Design review of the part built by this model. Coordinates are the model's own, in mm. Give positions to 0.01 mm unless a question says otherwise; leave off trailing zeros. Loops run counter-clockwise (first coordinate to the right, second up) from the corner with the lowest first, then second, coordinate; pieces in that order, holes last. Notation, with made-up numbers: M 4.5,24.5 L 55.5,24.5 A16 ccw 55.5,35.5 Z; hole C 10.5,61 d10. An arc over 180 degrees is marked long. Use a Markdown table: item, result. Add a question column.
(1) Insertion check: pin 1 Ø8 at (x, z) = (-42.5, -36.5) entering from +Y; pin 2 Ø8 at (y, z) = (-12.5, -1.5) entering from -X; pin 3 Ø4 at (y, z) = (-2, 41.5) entering from +X; pin 4 Ø5 at (x, z) = (-48, 65) entering from -Y. Each pin has a flat end and moves straight along its axis. Give the tip position at first contact, or say it passes through.
(2) For probe 1 along Z at (x, y) = (-10, -3); probe 2 along Z at (x, y) = (63, -2); probe 3 along X at (y, z) = (-17, -75), list the stretches that pass through material, from the lowest coordinate up.
(3) Add section C-C, the plane z = 24. Give the boundary of the cut face in (x, y), then the cut area to 3 significant figures.
(4) Add section A-A, the plane y = -20.25. Give the boundary of the cut face in (x, z), then the cut area to 3 significant figures.
(5) Add section D-D, the plane x = 24. Give the boundary of the cut face in (y, z).
```python
from build123d import *

# Parameters (mm, degrees)
SKETCH1_W            = 5.08
SKETCH1_H            = 5.08
BOSS_EXTRUDE2_DEPTH  = 5.08
BOSS_EXTRUDE7_DEPTH  = 5.08
BOSS_EXTRUDE8_DEPTH  = 1.27
BOSS_EXTRUDE9_DEPTH  = 12.7
BOSS_EXTRUDE10_DEPTH = 12.7
SKETCH1_5_W          = 5.08
SKETCH1_5_H          = 5.08
BOSS_EXTRUDE12_DEPTH = 25.4
BOSS_EXTRUDE13_DEPTH = 2.54
FILLET4_R            = 5.08


with BuildPart() as part:
    # Sketch1 → Boss-Extrude2 (new body)
    with BuildSketch(Plane(origin=(0, 0, 0), x_dir=(1, 0, 0), z_dir=(0, 1, 0))):
        Polygon((1.79979496, -9.735410081), (75.45979496, -9.735410081), (75.45979496, 85.514589919), (-19.79020504, 85.514589919), (-19.79020504, 34.079589919), (18.30979496, 34.079589919), (19.57979496, 34.079589919), (24.02479496, 34.079589919), (25.29479496, 34.079589919), (29.73979496, 34.079589919), (31.00979496, 34.079589919), (43.70979496, 34.079589919), (44.97979496, 34.079589919), (49.42479496, 34.079589919), (50.69479496, 34.079589919), (55.13979496, 34.079589919), (56.40979496, 34.079589919), (56.40979496, 21.379589919), (55.13979496, 21.379589919), (50.69479496, 21.379589919), (49.42479496, 21.379589919), (44.97979496, 21.379589919), (43.70979496, 21.379589919), (31.00979496, 21.379589919), (29.73979496, 21.379589919), (25.29479496, 21.379589919), (24.02479496, 21.379589919), (19.57979496, 21.379589919), (18.30979496, 21.379589919), (-19.79020504, 21.379589919), (-19.79020504, 11.854589919), (-30.58520504, 11.854589919), (-30.58520504, -28.571024106), (-30.58520504, -41.271024106), (-30.58520504, -42.755410081), (-30.58520504, -55.455410081), (-31.85520504, -55.455410081), (-36.30020504, -55.455410081), (-37.57020504, -55.455410081), (-42.01520504, -55.455410081), (-43.28520504, -55.455410081), (-43.28520504, -42.755410081), (-43.28520504, -41.271024106), (-43.28520504, -28.571024106), (-43.28520504, 11.854589919), (-74.40020504, 11.854589919), (-74.40020504, -83.395410081), (1.79979496, -83.395410081), align=None)
        with Locations((-7.72520504, 2.329589919)):
            Rectangle(SKETCH1_W, SKETCH1_H, mode=Mode.SUBTRACT)
        with Locations((-7.72520504, 75.989589919)):
            Rectangle(SKETCH1_W, SKETCH1_H, mode=Mode.SUBTRACT)
        with Locations((65.942961522, 75.973256793)):
            Rectangle(SKETCH1_W, SKETCH1_H, mode=Mode.SUBTRACT)
    extrude(amount=-BOSS_EXTRUDE2_DEPTH)

    # Sketch4 → Boss-Extrude7 (add)
    with BuildSketch(Plane(origin=(0, 0, 0), x_dir=(1, 0, 0), z_dir=(0, 1, 0))):
        Polygon((-46.46020504, 11.854589919), (-43.28520504, 11.854589919), (-43.28520504, 34.079589919), (-19.79020504, 34.079589919), (-19.79020504, 37.254589919), (-46.46020504, 37.254589919), align=None)
    extrude(amount=-BOSS_EXTRUDE7_DEPTH)



with BuildPart() as body_2:
    # Sketch4<5> → Boss-Extrude8 (new body)
    with BuildSketch(Plane(origin=(0, 0, 0), x_dir=(1, 0, 0), z_dir=(0, 1, 0))):
        Polygon((-30.58520504, 11.854589919), (-19.79020504, 11.854589919), (-19.79020504, 21.379589919), (-19.79020504, 34.079589919), (-43.28520504, 34.079589919), (-43.28520504, 11.854589919), align=None)
    extrude(amount=-BOSS_EXTRUDE8_DEPTH)


with BuildPart() as part_1:
    add(part.part)

    add(body_2.part)  # Boss-Extrude9 merges body 2
    # Sketch5 → Boss-Extrude9 (add)
    with BuildSketch(Plane.ZY.offset(30.58520504)):
        Polygon((55.455410081, -5.08), (55.455410081, 0), (-11.854589919, 0), (-11.854589919, -1.279733849), align=None)
    extrude(amount=BOSS_EXTRUDE9_DEPTH)

    # Sketch6 → Boss-Extrude10 (add)
    with BuildSketch(Plane.XY.offset(-34.079589919)):
        Polygon((56.40979496, -5.08), (56.40979496, 0), (-19.79020504, 0), (-19.79020504, -1.27), align=None)
    extrude(amount=BOSS_EXTRUDE10_DEPTH)

    # Sketch1<5> → Boss-Extrude12 (add)
    with BuildSketch(Plane(origin=(0, 0, 0), x_dir=(1, 0, 0), z_dir=(0, 1, 0))):
        with Locations((-7.72520504, 75.989589919)):
            Rectangle(SKETCH1_5_W, SKETCH1_5_H)
        with Locations((65.942961522, 75.973256793)):
            Rectangle(SKETCH1_5_W, SKETCH1_5_H)
        with Locations((-7.72520504, 2.329589919)):
            Rectangle(SKETCH1_5_W, SKETCH1_5_H)
    extrude(amount=-BOSS_EXTRUDE12_DEPTH)

    # Sketch7 → Boss-Extrude13 (add)
    with BuildSketch(Plane.XZ.offset(5.08)):
        Polygon((-74.40020504, -11.854589919), (-46.46020504, -11.854589919), (-46.46020504, -37.254589919), (-19.79020504, -37.254589919), (-19.79020504, -85.514589919), (75.45979496, -85.514589919), (75.45979496, 9.735410081), (1.79979496, 9.735410081), (1.79979496, 83.395410081), (-74.40020504, 83.395410081), align=None)
        Polygon((-30.58520504, 55.455410081), (-43.28520504, 55.455410081), (-43.28520504, -34.079589919), (56.40979496, -34.079589919), (56.40979496, -21.379589919), (-19.79020504, -21.379589919), (-19.79020504, -11.854589919), (-30.58520504, -11.854589919), align=None, mode=Mode.SUBTRACT)
    extrude(amount=BOSS_EXTRUDE13_DEPTH)

    # Fillet4
    fillet4_edges = [part_1.edges().sort_by_distance(p)[0] for p in [
        (-43.28520504, -4.445, -34.079589919),
        (-46.46020504, -3.81, -37.254589919),
        (-19.79020504, -4.445, -11.854589919),
    ]]
    fillet(fillet4_edges, radius=FILLET4_R)


solid = part_1.part
```
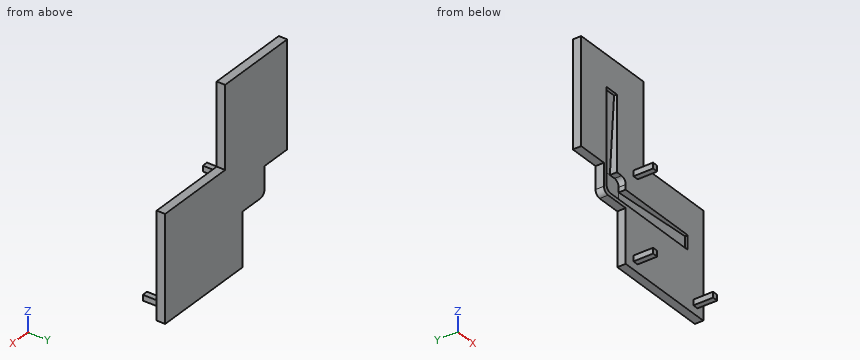
Established:
| question | item | result |
|---|---|---|
| 1 | pin 1 | y = 0 |
| 1 | pin 2 | x = -10.27 |
| 1 | pin 3 | x = 1.8 |
| 1 | pin 4 | y = -7.62 |
| 2 | probe 1 | -85.51 to -34.08, -21.38 to 83.4 |
| 2 | probe 2 | -85.51 to 9.74 |
| 2 | probe 3 | -10.27 to -5.19, 63.4 to 68.48 |
| 3 | outline | M -74.4,-7.62 L -43.29,-7.62 L -43.29,-3.3 L -30.59,-3.3 L -30.59,-7.62 L 1.8,-7.62 L 1.8,0 L -74.4,0 Z |
| 3 | area | 526 mm^2 |
| 4 | outline | M -10.27,-78.53 L -5.19,-78.53 L -5.19,-73.45 L -10.27,-73.45 Z; M -10.27,-4.87 L -5.19,-4.87 L -5.19,0.21 L -10.27,0.21 Z; M 63.4,-78.51 L 68.48,-78.51 L 68.48,-73.43 L 63.4,-73.43 Z |
| 4 | area | 77.4 mm^2 |
| 5 | outline | M -7.62,-85.51 L 0,-85.51 L 0,9.74 L -7.62,9.74 L -7.62,-21.38 L -3.46,-21.38 L -3.46,-34.08 L -7.62,-34.08 Z |
